```python
from build123d import *

# Parameters (mm, degrees)
BOSS_EXTRUDE2_DEPTH      = 152.4
BOSS_EXTRUDE2_DEPTH_BACK = 152.4
SKETCH3_R                = 6
SKETCH3_R_2              = 5
CUT_EXTRUDE1_DEPTH       = 153.636037684
CUT_EXTRUDE1_DEPTH_BACK  = 153.636037684
SKETCH4_R                = 1.524
SKETCH5_R                = 6
CUT_EXTRUDE2_DEPTH       = 234.8


with BuildPart() as part:
    # Sketch3 → Boss-Extrude2 (new, two sides: drawn at the far end of the back side and taken through both)
    with BuildSketch(Plane.XY.offset(-BOSS_EXTRUDE2_DEPTH_BACK)):
        with Locations(Location((0, 0, 0), (0, 0, 180))):
            Circle(SKETCH3_R)
        with Locations(Location((0, 0, 0), (0, 0, 180))):
            Circle(SKETCH3_R_2, mode=Mode.SUBTRACT)
    extrude(amount=BOSS_EXTRUDE2_DEPTH + BOSS_EXTRUDE2_DEPTH_BACK)

    # Sketch4 → Cut-Extrude1 (cut, two sides: drawn at the far end of the back side and taken through both)
    with BuildSketch(Plane(origin=(0, 0, 0), x_dir=(1, 0, 0), z_dir=(0, 1, 0)).offset(-CUT_EXTRUDE1_DEPTH_BACK)):
        with Locations(Location((0, -147.82, 0), (0, 0, 270))):
            Circle(SKETCH4_R)
    extrude(amount=CUT_EXTRUDE1_DEPTH + CUT_EXTRUDE1_DEPTH_BACK, mode=Mode.SUBTRACT)

    # Sketch5 → Cut-Extrude2 (cut)
    with BuildSketch(Plane(origin=(0, 0, -152.4), x_dir=(-1, 0, 0), z_dir=(0, 0, -1))):
        with Locations(Location((0, 0, 0), (0, 0, 180))):
            Circle(SKETCH5_R)
    extrude(amount=-CUT_EXTRUDE2_DEPTH, mode=Mode.SUBTRACT)


solid = part.part
```
The model under review builds one solid part; all positions refer to its coordinate system, in mm. Round coordinates to 2 decimals unless told otherwise and drop trailing zeros. Loops run counter-clockwise (first coordinate to the right, second up) from the corner with the lowest first, then second, coordinate; pieces in that order, holes last. Notation, with made-up numbers: M 52.25,73.25 L 60.25,73.25 A21 cw 60.25,98.25 Z; hole C 19,53.5 d11. An arc over 180 degrees is marked long. Put each result on its own line as item: value.
Q1. Consider section A-A, the plane x = 0. Give the boundary of the cut face in (y, z), then the cut area to 3 significant figures.
Result set:
outline: M -6,82.4 L -5,82.4 L -5,146.3 L -6,146.3 Z; M -6,149.34 L -5,149.34 L -5,152.4 L -6,152.4 Z; M 5,82.4 L 6,82.4 L 6,146.3 L 5,146.3 Z; M 5,149.34 L 6,149.34 L 6,152.4 L 5,152.4 Z
area: 134 mm²
Q2. Mouldability with a two-part tool opening along X and no side actions: class faces 1 (the cylindrical face through (-5.54, 2.3, 116.91)), 2 (the cylindrical face through (-0.58, -5.39, 149.23)), 3 (the cylindrical face through (-1.488, 5.375, 147.49)), 4 (the flat face through (4, -4, 152.4)) as released by +X, released by -X, zero draft, split by the parting line, or undercut.
Result set:
face 1: split by the parting line
face 2: undercut
face 3: undercut
face 4: zero draft
Q3. Consider section D-D, the plane z = 139.5. Give the boundary of the cut face in (x, y).
Result set:
outline: C 0,0 d12; hole C 0,0 d10
Q4. For pin 1 (3 mm diameter, centred on x = 2, y = 0.5, fed in from +Z); pin 2 (1.5 mm diameter, centred on y = -3, z = 102.5, fed in from -X); pin 3 (3 mm diameter, centred on y = 2, z = 121.5, fed in from -X), all flat-tipped, find the tip position at first contact; note any pin that passes through.
Result set:
pin 1: passes through
pin 2: stops at x = -5.56
pin 3: stops at x = -5.98
Q5. Consider section B-B, the plane y = 0. Give the boundary of the cut face in (x, z).
Result set:
outline: M -6,82.4 L -5,82.4 L -5,152.4 L -6,152.4 Z; M 5,82.4 L 6,82.4 L 6,152.4 L 5,152.4 Z
Q6. Consider section C-C, the plane z = 147.82. Give the boundary of the cut face in (x, y).
Result set:
outline: M -1.52,-5.8 L -1.52,-4.76 A5 cw -1.52,4.76 L -1.52,5.8 A6 ccw Z; M 1.52,-5.8 A6 ccw 1.52,5.8 L 1.52,4.76 A5 cw 1.52,-4.76 Z
Q7. To check wall thickness, follow L1, parallel to Y at x = 0, z = 113; L2, parallel to X at y = 0.25, z = 144; L3, parallel to Z at x = 0, y = -5.5. State the ranges of each line that lie inside material, in increasing order.
Result set:
L1: y = -6 to -5, 5 to 6
L2: x = -5.99 to -4.99, 4.99 to 5.99
L3: z = 82.4 to 146.3, 149.34 to 152.4
